CAD build for the part. Positions are in the model's coordinates, mm. Face numbers are marked on the shaded views. A direction names the side the tool comes from. Coordinates: 2 decimals unless noted, no trailing zeros. Loops run counter-clockwise (first coordinate to the right, second up) from the corner with the lowest first, then second, coordinate; pieces in that order, holes last.
1) Saw through at B-B, the plane z = -11.5. Write the cut outline in (x, y), and give its area (3 significant figures).
2) Wall check: line 1 along Z through (x, y) = (-36, 8); line 2 along X through (y, z) = (0, 21.5); line 3 along Z through (x, y) = (-46.5, 4). Give the ranges that are in metal, low to high.
3) Pin check, flat tips, straight feed: pin 1 Ø8 at (x, z) = (-51, -15.5) entering from +Y; pin 2 Ø5 at (x, y) = (-73.5, -1.5) entering from +Z; pin 3 Ø4 at (y, z) = (-9, 8.5) entering from +X. Stop position of each tip, or through.
4) Which spindle directions (+Z, -Z, +X, -X, +Y, -Y) get a long thin tool onto all of the face, cutting with end or side? Do the marked faces 1, 2 and 3. Say none if no direction does.
5) Saw through at C-C, the plane x = -103.5. Write the cut outline in (y, z).
6) Saw through at A-A, the plane y = 0. Write the cut outline in (x, z), and give its area (3 significant figures).
7) Saw through at D-D, the plane z = 9. Write the cut outline in (x, y), and give its area (3 significant figures).
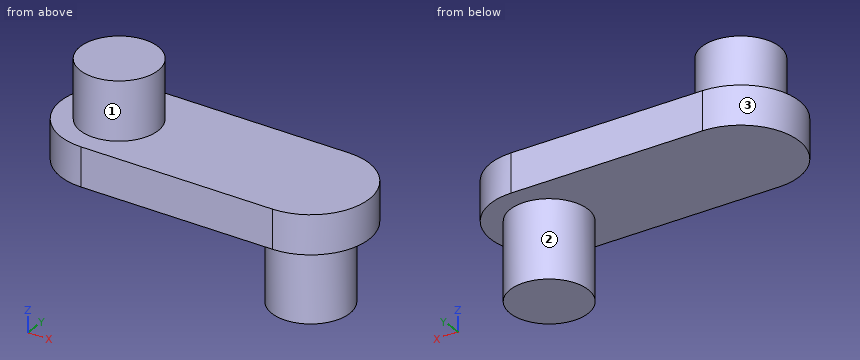
```python
from build123d import *

# Parameters (mm, degrees)
SKETCH1_R           = 10
BOSS_EXTRUDE1_DEPTH = 10
BOSS_EXTRUDE2_START = -30
SKETCH2_R           = 10
BOSS_EXTRUDE2_DEPTH = 30
SKETCH3_R           = 10
BOSS_EXTRUDE3_DEPTH = 25


with BuildPart() as part:
    # Sketch1 → Boss-Extrude1 (new body)
    with BuildSketch(Plane.XY):
        with BuildLine():
            Line((-95.01107872, 15), (-45.01107872, 15))
            ThreePointArc((-45.01107872, 15), (-30.01107872, 0), (-45.01107872, -15))
            Line((-45.01107872, -15), (-95.01107872, -15))
            ThreePointArc((-95.01107872, -15), (-110.01107872, 0), (-95.01107872, 15))
        make_face()
        with Locations((-95.01107872, 0)):
            Circle(SKETCH1_R, mode=Mode.SUBTRACT)
        with Locations((-45.01107872, 0)):
            Circle(SKETCH1_R, mode=Mode.SUBTRACT)
    extrude(amount=BOSS_EXTRUDE1_DEPTH)

    # Sketch2 → Boss-Extrude2 (add)
    with BuildSketch(Plane.XY.offset(10).offset(BOSS_EXTRUDE2_START)):
        with Locations((-45.01107872, 0)):
            Circle(SKETCH2_R)
    extrude(amount=BOSS_EXTRUDE2_DEPTH)

    # Sketch3 → Boss-Extrude3 (add)
    with BuildSketch(Plane(origin=(0, 0, 0), x_dir=(-1, 0, 0), z_dir=(0, 0, -1))):
        with Locations((95.01107872, 0)):
            Circle(SKETCH3_R)
    extrude(amount=-BOSS_EXTRUDE3_DEPTH)


solid = part.part
```
Data:
1. outline: circle Ø20 at (-45.01, 0)
1. area: 314 mm2
2. line 1: z = 0 to 10
2. line 2: x = -105.01 to -85.01
2. line 3: z = -20 to 10
3. pin 1: stops at y = 9.8
3. pin 2: stops at z = 10
3. pin 3: stops at x = -31.74
4. face 1: +Z
4. face 2: -Z
4. face 3: +Z, -Z, -X
5. outline: (-12.37, 0) - (12.37, 0) - (12.37, 10) - (5.29, 10) - (5.29, 25) - (-5.29, 25) - (-5.29, 10) - (-12.37, 10) - close
6. outline: (-110.01, 0) - (-55.01, 0) - (-55.01, -20) - (-35.01, -20) - (-35.01, 0) - (-30.01, 0) - (-30.01, 10) - (-85.01, 10) - (-85.01, 25) - (-105.01, 25) - (-105.01, 10) - (-110.01, 10) - close
6. area: 1,500 mm2
7. outline: (-95.01, -15) - (-45.01, -15) arc R15 ccw to (-45.01, 15) - (-95.01, 15) arc R15 ccw to start
7. area: 2,210 mm2
